Geometry check sheet. Reference: drawing and pictorial views, mm from the part's lowest x, y, z. Give positions to 0.01 mm unless a question says otherwise; leave off trailing zeros. Loops run counter-clockwise (first coordinate to the right, second up) from the corner with the lowest first, then second, coordinate; pieces in that order, holes last. Notation, with made-up numbers: M 31.5,-12.75 L 65.5,-12.75 A22 cw 65.5,26.25 Z; hole C 7.5,-26.75 d4. An arc over 180 degrees is marked long. Put each result on its own line as item: value. Start each with the question number.
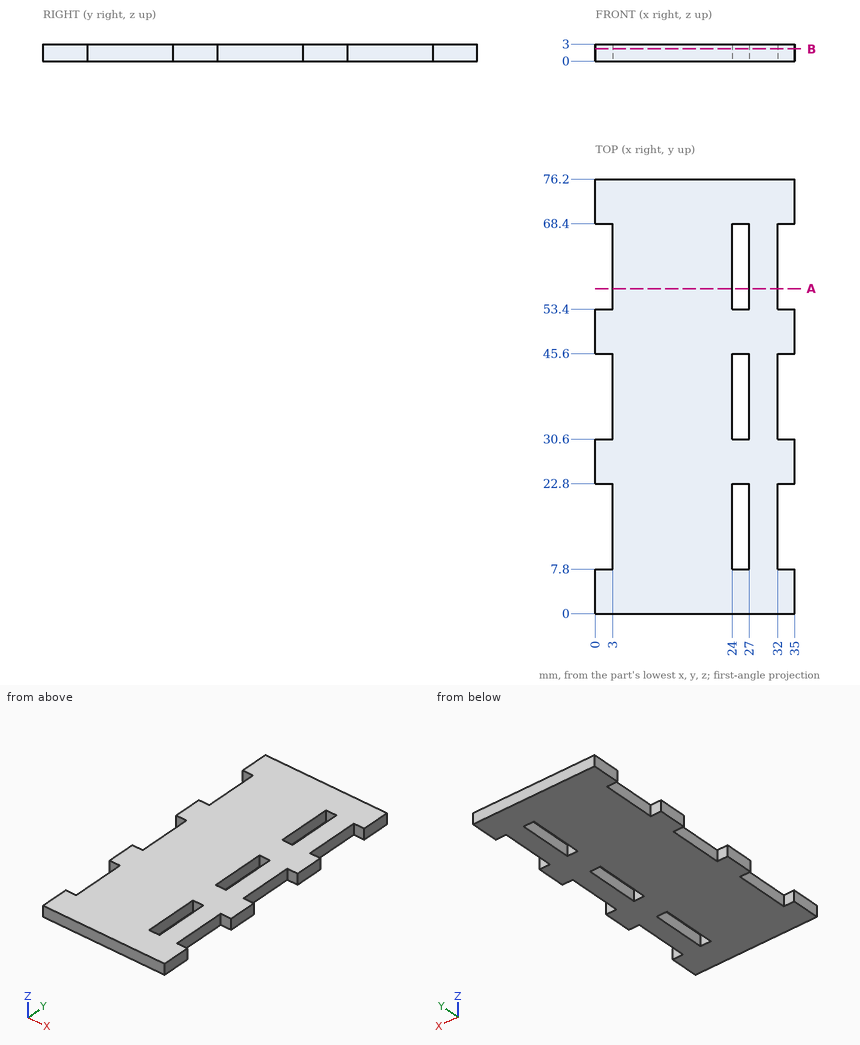
Q1. Section check A-A, the plane y = 57. Record the cut outline in (x, z), then the cut area to 3 significant figures.
Q2. Section check B-B, the plane z = 2.15. Give the number of separate pieces and of enclosed holes in the cut face, then the cut area to 3 significant figures.
Q3. Thickness scan on line 1 along Y through (x, z) = (24.5, 0.65); line 2 along X through (y, z) = (9, 0.3). Record the ranges inside material, lowest first. Write a range as [from, to].
Q4. Depth check by flat-ended pin: P1, Ø0.9, axis at y = 37.5, z = 1, coming from the +X side; P2, Ø1.5, axis at y = 59, z = 2, coming from the -X side. Enter the tip coordinate at first touch or a pass-through.
Found:
1. outline: M 3,0 L 24,0 L 24,3 L 3,3 Z; M 27,0 L 32,0 L 32,3 L 27,3 Z
1. area: 78.0 mm^2
2. separate pieces: 1
2. enclosed holes: 3
2. area: 2,260 mm^2
3. line 1: y = [0, 7.8], [22.8, 30.6], [45.6, 53.4], [68.4, 76.2]
3. line 2: x = [3, 24], [27, 32]
4. P1: stops at x = 32
4. P2: stops at x = 3
